Study the drawing (mm; zero at the part's minimum x, y, z) and answer. A direction names the side the tool comes from. Coordinates: 2 decimals unless noted, no trailing zeros. Write each loop counter-clockwise with the first axis right and the second up, starting at its lowest first coordinate (ties: lowest second). Pieces come first, ordered by that corner, then holes. Notation, with made-up numbers: M -5.75,11 L 48.25,11 A25 ccw 48.25,48 Z; hole C 14.5,21 d5. An arc over 180 degrees is marked long. Answer as a JSON object with one key per item and string values. Group by question number.
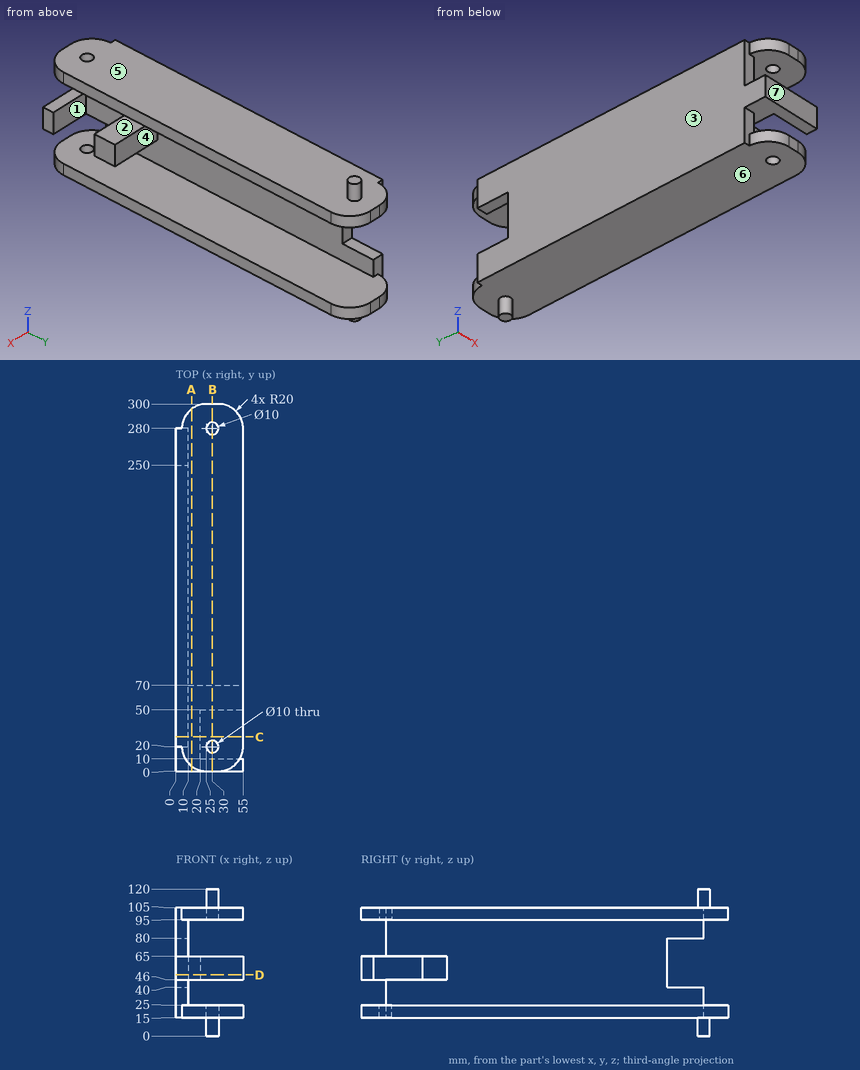
Item 1: For a pull along Z with two mould halves and no side action, classify the marked faces 4, 5, 6 and 7 as +Z half, -Z half, draft (parallel to the pull), parting line (faces both ways), or undercut.
Item 2: A cutting plane is placed at D-D, the plane z = 50. Write down the section's boundary in (x, y).
Item 3: A tool of negligible diameter and unlimited length cuts with its end or side. For the marked faces 1, 2 and 3, from which of +Z, -Z, +X, -X, +Y, -Y can it reach the whole face along a straight path? Write none if from no direction.
Item 4: Consider L1, parallel to Z at x = 30, y = 62.5; L2, parallel to Y at x = 30, z = 22; L3, parallel to Z at x = 14, y = 204. Determine where each line is inside the solid, lowest interval first. Write a range as from..to.
Item 5: Flat-ended cylindrical pins translate along their axes: pin 1 Ø21 at (x, z) = (43, 56) entering from +Y; pin 2 Ø1 at (x, y) = (8, 245) entering from +Z; pin 3 Ø1 at (x, y) = (38.5, 221.5) entering from -Z. Find the tip coordinate at first contact, or state that the pin passes through.
Item 6: A cutting plane is placed at A-A, the plane x = 13. Write down the section's boundary in (y, z), and give its area (3 significant figures).
Item 7: A cutting plane is placed at B-B, the plane x = 30. State how many separate pieces and enclosed holes the cut face has, and give its area (3 significant figures).
Item 8: A cutting plane is placed at C-C, the plane y = 28. Write down the section's boundary in (x, z), and give its area (3 significant figures).
Answer:
{
 "1": {"face 4": "undercut", "face 5": "+Z half", "face 6": "-Z half", "face 7": "draft"},
 "2": {"outline": "M 0,0 L 55,0 L 55,10 L 20,10 L 20,50 L 55,50 L 55,70 L 10,70 L 10,250 L 0,250 Z"},
 "3": {"face 1": "+X", "face 2": "+X, -Y", "face 3": "+Z, -Z, -X, +Y, -Y"},
 "4": {"L1": "15..25, 46..65, 95..105", "L2": "0..15, 25..300", "L3": "15..25, 95..105"},
 "5": {"pin 1": "y = 70", "pin 2": "z = 105", "pin 3": "z = 15"},
 "6": {"outline": "M 0,46 L 70,46 L 70,65 L 0,65 Z; M 4,15 L 296,15 L 296,25 L 4,25 Z; M 4,95 L 296,95 L 296,105 L 4,105 Z", "area": "7,170 mm2"},
 "7": {"separate pieces": "6", "enclosed holes": "0", "area": "6,670 mm2"},
 "8": {"outline": "M 0,15 L 55,15 L 55,25 L 10,25 L 10,46 L 20,46 L 20,65 L 10,65 L 10,95 L 55,95 L 55,105 L 0,105 Z", "area": "1,990 mm2"}
}
